The drawing under review shows one solid part. Ordinate dimensions are in mm from its lowest x, y, z. Round coordinates to 2 decimals unless told otherwise and drop trailing zeros. Loops run counter-clockwise (first coordinate to the right, second up) from the corner with the lowest first, then second, coordinate; pieces in that order, holes last. Notation, with made-up numbers: (63.5, 52) -> (121.5, 52) arc R19 ccw to (121.5, 84) -> close; hole circle Ø9 at (-7, 4.25). An arc over 180 degrees is marked (long way). Answer as CSV lines item,"result". Start each with the question number.
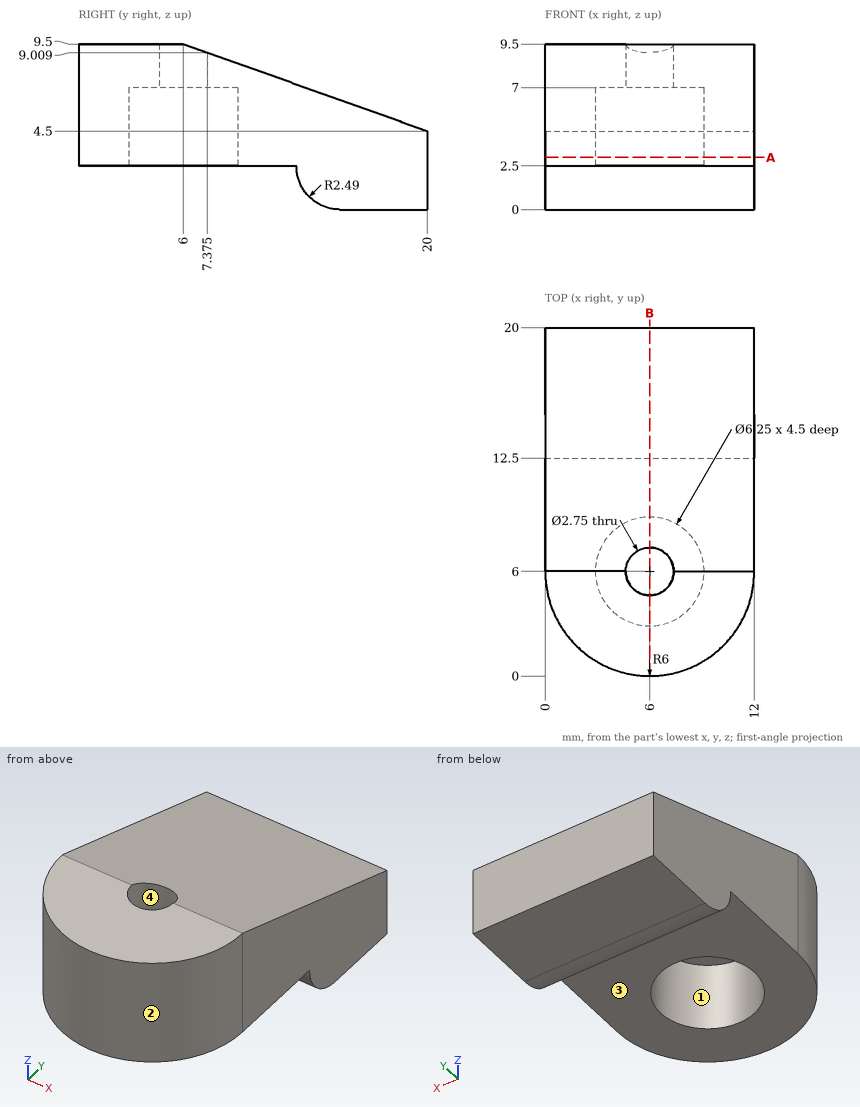
Q1. For pin 1 Ø1 at (x, y) = (9, 10.5) entering from -Z; pin 2 Ø2 at (x, z) = (2, 4.5) entering from -Y; pin 3 Ø1 at (y, z) = (2, 2.5) entering from -X, all flat-tipped, find the tip position at first contact; note any pin that passes through.
Q2. Add section B-B, the plane x = 6. Give the boundary of the cut face in (y, z) (3 decimals).
Q3. To check wall thickness, follow probe 1 along Y at (x, z) = (6, 4) (3 decimals); probe 2 along X at (y, z) = (6, 8.05) (3 decimals); probe 3 along Z at (x, y) = (4, 5.75). State the ranges of each line that lie inside material, in increasing order. Write a range as from..to.
Q4. Mouldability with a two-part tool opening along Y and no side actions: class the marked faces 1, 2, 3 and 4 as pulls with the +Y half, pulls with the -Y half, needs draft (parallel to the pull), parting line crosses it, or undercut.
Q5. Add section A-A, the plane z = 3. Give the boundary of the cut face in (x, y) (3 decimals).
Worked answers:
1,pin 1,"stops at z = 2.5"
1,pin 2,"stops at y = 0.8"
1,pin 3,"stops at x = 1.13"
2,outline,"(0, 2.5) -> (2.875, 2.5) -> (2.875, 7) -> (4.625, 7) -> (4.625, 9.5) -> (0, 9.5) -> close; (7.375, 7) -> (9.125, 7) -> (9.125, 2.5) -> (12.5, 2.5) -> (12.5, 2.49) arc R2.49 ccw to (14.99, 0) -> (20, 0) -> (20, 4.5) -> (7.375, 9.009) -> close"
3,probe 1,"y = 0..2.875, 9.125..20"
3,probe 2,"x = 0..4.625, 7.375..12"
3,probe 3,"z = 7..9.5"
4,face 1,"undercut"
4,face 2,"pulls with the -Y half"
4,face 3,"needs draft"
4,face 4,"undercut"
5,outline,"(0, 6) arc R6 ccw to (12, 6) -> (12, 20) -> (0, 20) -> close; hole circle Ø6.25 at (6, 6)"
